from build123d import *

# Parameters (mm, degrees)
SKETCH1_W           = 61
SKETCH1_H           = 61
SKETCH1_W_2         = 57
SKETCH1_H_2         = 57
BOSS_EXTRUDE2_DEPTH = 30
SKETCH2_W           = 58.6
SKETCH2_H           = 58.6
CUT_EXTRUDE1_DEPTH  = 3.2
SKETCH4_RX          = 3
SKETCH4_RY          = 2.5
CUT_EXTRUDE2_DEPTH  = 73.878323252


with BuildPart() as part:
    # Sketch1 → Boss-Extrude2 (new body)
    with BuildSketch(Plane(origin=(0, 0, 0), x_dir=(1, 0, 0), z_dir=(0, 1, 0))):
        with Locations((0, 28.5)):
            Rectangle(SKETCH1_W, SKETCH1_H)
        with Locations((0, 28.5)):
            Rectangle(SKETCH1_W_2, SKETCH1_H_2, mode=Mode.SUBTRACT)
    extrude(amount=BOSS_EXTRUDE2_DEPTH)

    # Sketch2 → Cut-Extrude1 (cut)
    with BuildSketch(Plane(origin=(0, 30, 0), x_dir=(1, 0, 0), z_dir=(0, 1, 0))):
        with Locations((0, 28.5)):
            Rectangle(SKETCH2_W, SKETCH2_H)
    extrude(amount=-CUT_EXTRUDE1_DEPTH, mode=Mode.SUBTRACT)

    # Sketch4 → Cut-Extrude2 (cut, through all)
    with BuildSketch(Plane(origin=(0, 0, 0), x_dir=(-1, 0, 0), z_dir=(0, 0, -1))):
        with BuildLine():
            Line((-5.98277454, 23.2), (-5.98277454, 25.8))
            Line((-5.98277454, 25.8), (-8.131556664, 25.8))
            ThreePointArc((-8.131556664, 25.8), (-8.523646049, 25.719927124), (-8.852943985, 25.492531828))
            Line((-8.852943985, 25.492531828), (-9.479161861, 24.840221541))
            ThreePointArc((-9.479161861, 24.840221541), (-9.685510311, 24.520927357), (-9.75777454, 24.147689712))
            Line((-9.75777454, 24.147689712), (-9.75777454, 23.6))
            ThreePointArc((-9.75777454, 23.6), (-9.640617252, 23.317157288), (-9.35777454, 23.2))
            Line((-9.35777454, 23.2), (-5.98277454, 23.2))
        make_face()
        with BuildLine():
            Line((-3.833992416, 25.8), (-5.98277454, 25.8))
            Line((-5.98277454, 25.8), (-5.98277454, 23.2))
            Line((-5.98277454, 23.2), (-2.60777454, 23.2))
            ThreePointArc((-2.60777454, 23.2), (-2.324931828, 23.317157288), (-2.20777454, 23.6))
            Line((-2.20777454, 23.6), (-2.20777454, 24.147689712))
            ThreePointArc((-2.20777454, 24.147689712), (-2.280038769, 24.520927357), (-2.486387219, 24.840221541))
            Line((-2.486387219, 24.840221541), (-3.112605095, 25.492531828))
            ThreePointArc((-3.112605095, 25.492531828), (-3.441903031, 25.719927124), (-3.833992416, 25.8))
        make_face()
        with Locations(Location((5.992555786, 23.215339324), (0, 0, 180))):
            Ellipse(SKETCH4_RX, SKETCH4_RY)
    extrude(amount=-CUT_EXTRUDE2_DEPTH, mode=Mode.SUBTRACT)


solid = part.part
The listing builds one solid part. Answer for the finished solid, in the listing's coordinates (mm). A direction names the side the tool comes from. Give positions to 0.01 mm unless a question says otherwise; leave off trailing zeros. Write each loop counter-clockwise with the first axis right and the second up, starting at its lowest first coordinate (ties: lowest second). Pieces come first, ordered by that corner, then holes. Notation, with made-up numbers: (36.5, 23) - (65.5, 23) arc R30 ccw to (65.5, 59) - close; hole circle Ø2 at (41, -15). An arc over 180 degrees is marked (long way). One line per question, with ' | ' between items. Start each with the question number.
1. Section A-A, the plane z = -11 is taken. Determine the outline of the cut face in (x, y), then the cut area to 3 significant figures.
2. Section D-D, the plane x = -7 is taken. Count the separate pieces of the cut face and the enclosed holes in it, then the cut area to 3 significant figures.
3. Section C-C, the plane y = 9.5 is taken. Determine the outline of the cut face in (x, z), then the cut area to 3 significant figures.
4. For faces 1 (the face through (-28.5, 13, -28)), 2 (the face through (29.3, 28, -28)), 3 (the face through (6, 25.8, 1)), determine the directions among +Z, -Z, +X, -X, +Y, -Y from which every point of the face is accessible in a straight line to the end or side of a thin tool.
5. Straight lines are drawn through the part: line 1 (X direction, y = 2, z = -32); line 2 (Z direction, x = -16.5, y = 19); line 3 (X direction, y = 28, z = -21.5). For each, find the intervals that lie inside material, in ascending order.
6. Section B-B, the plane x = -17 is taken. Determine the outline of the cut face in (y, z), then the cut area to 3 significant figures.
7. Determine the mould class of faces 4 (the face through (-2, 0, 1)), 5 (the face through (30.5, 15, -28)), 6 (the face through (0, 13, 0)), 7 (the face through (6, 23.2, 1)) for opening direction X: +X half, -X half, draft (parallel to the pull), parting line (faces both ways), or undercut.
Result:
1) outline: (-30.5, 0) - (-28.5, 0) - (-28.5, 26.8) - (-29.3, 26.8) - (-29.3, 30) - (-30.5, 30) - close; (28.5, 0) - (30.5, 0) - (30.5, 30) - (29.3, 30) - (29.3, 26.8) - (28.5, 26.8) - close | area: 115 mm2
2) separate pieces: 3 | enclosed holes: 0 | area: 105 mm2
3) outline: (-30.5, -59) - (30.5, -59) - (30.5, 2) - (-30.5, 2) - close; hole (-28.5, -57) - (28.5, -57) - (28.5, 0) - (-28.5, 0) - close | area: 472 mm2
4) face 1: +Y, -Y | face 2: +Y | face 3: +Z
5) line 1: x = -30.5 to -28.5, 28.5 to 30.5 | line 2: z = -59 to -57, 0 to 2 | line 3: x = -30.5 to -29.3, 29.3 to 30.5
6) outline: (0, -59) - (30, -59) - (30, -57.8) - (26.8, -57.8) - (26.8, -57) - (0, -57) - close; (0, 0) - (26.8, 0) - (26.8, 0.8) - (30, 0.8) - (30, 2) - (0, 2) - close | area: 115 mm2
7) face 4: draft | face 5: +X half | face 6: undercut | face 7: undercut
